```python
from build123d import *

# Parameters (mm, degrees)
SKETCH3_R          = 6.5
SKETCH3_W          = 8
SKETCH3_H          = 8
CUT_EXTRUDE1_DEPTH = 3


with BuildPart() as part:
    # Sketch1 → Revolve1 (revolve)
    with BuildSketch(Plane.XY):
        with BuildLine():
            Line((-2.5, -5), (-2.5, 1))
            ThreePointArc((-2.5, 1), (-4.5, 3), (-6.5, 1))
            Line((-6.5, 1), (-6.5, -5))
            Line((-6.5, -5), (-2.5, -5))
        make_face()
    revolve(axis=Axis((0, 0, 0), (0, -1, 0)))

    # Sketch3 → Cut-Extrude1 (cut)
    with BuildSketch(Plane(origin=(0, -3, 0), x_dir=(-1, 0, 0), z_dir=(0, -1, 0))):
        Circle(SKETCH3_R)
        Rectangle(SKETCH3_W, SKETCH3_H, mode=Mode.SUBTRACT)
    extrude(amount=-CUT_EXTRUDE1_DEPTH, mode=Mode.SUBTRACT)


solid = part.part
```
The listing builds one solid part. Answer for the finished solid, in the listing's coordinates (mm). A direction names the side the tool comes from. Give positions to 0.01 mm unless a question says otherwise; leave off trailing zeros. Loops run counter-clockwise (first coordinate to the right, second up) from the corner with the lowest first, then second, coordinate; pieces in that order, holes last. Notation, with made-up numbers: (59.25, 74.25) - (90.25, 74.25) arc R15 ccw to (90.25, 86.25) - close; hole circle Ø11 at (52.5, -29). An arc over 180 degrees is marked (long way). Return JSON: item names as keys, results as strings. Group by question number.
1. Determine the mould class of faces 5 (the cylindrical face through (5.158, 0.493, 3.955)), 6 (the flat face through (-3, -5, 0)), 7 (the flat face through (4, -2, 0)) for opening direction Y: pulls with the +Y half, pulls with the -Y half, needs draft (parallel to the pull), parting line crosses it, or undercut.
2. Find section C-C (y = -1.75). Write down the section's boundary in (x, z), then the cut area to 3 significant figures.
3. Find section D-D (y = -3.5). Write down the section's boundary in (x, z), then the cut area to 3 significant figures.
4. Find section B-B (z = 0). Write down the section's boundary in (x, y).
5. Which of the six approach directions +Z, -Z, +X, -X, +Y, -Y give full straight-line access (tool end or side, diameter ignored) to faces 1 (the flat face through (0, -2, 4)), 2 (the flat face through (0, -2, -4)), 3 (the flat face through (-4, -2, 0)), 4 (the flat face through (0.1, -3, 4.2))?
6. Straight lines are drawn through the part: line 1 (Z direction, x = 0, y = -0.65); line 2 (Z direction, x = 0, y = -3.4). For each, find the intervals that lie inside material, in ascending order. Write a range as [from, to].
7. Find section A-A (x = 0). Write down the section's boundary in (y, z), then the cut area to 3 significant figures.
8. Given pin 1 Ø4 at (x, z) = (2, 0.5) entering from +Y; pin 2 Ø2.5 at (y, z) = (-1.5, 0) entering from +X; pin 3 Ø6.5 at (x, z) = (0, 0) entering from +Y; pin 4 Ø3.5 at (x, y) = (-0.5, -1.5) entering from -Z, each flat-ended and moving along its own axis, determine where each tip first touches the part or whether it passes through.
Verdict:
{
 "1": {"face 5": "needs draft", "face 6": "pulls with the -Y half", "face 7": "undercut"},
 "2": {"outline": "(-4, -4) - (4, -4) - (4, 4) - (-4, 4) - close; hole circle Ø5 at (0, 0)", "area": "44.4 mm^2"},
 "3": {"outline": "circle Ø13 at (0, 0); hole circle Ø5 at (0, 0)", "area": "113 mm^2"},
 "4": {"outline": "(-6.5, -5) - (-2.5, -5) - (-2.5, 1) arc R2 ccw to (-6.5, 1) - (-6.5, 0) - (-4, 0) - (-4, -3) - (-6.5, -3) - close; (2.5, -5) - (6.5, -5) - (6.5, -3) - (4, -3) - (4, 0) - (6.5, 0) - (6.5, 1) arc R2 ccw to (2.5, 1) - close"},
 "5": {"face 1": "+Z, +X, -X", "face 2": "-Z, +X, -X", "face 3": "+Z, -Z, -X", "face 4": "none"},
 "6": {"line 1": "z = [-4, -2.5], [2.5, 4]", "line 2": "z = [-6.5, -2.5], [2.5, 6.5]"},
 "7": {"outline": "(-5, -6.5) - (-3, -6.5) - (-3, -4) - (0, -4) - (0, -6.5) - (1, -6.5) arc R2 ccw to (1, -2.5) - (-5, -2.5) - close; (-5, 2.5) - (1, 2.5) arc R2 ccw to (1, 6.5) - (0, 6.5) - (0, 4) - (-3, 4) - (-3, 6.5) - (-5, 6.5) - close", "area": "45.6 mm^2"},
 "8": {"pin 1": "stops at y = 2.95", "pin 2": "stops at x = 4", "pin 3": "stops at y = 2.56", "pin 4": "stops at z = -6.5"}
}
